```python
from build123d import *

# Parameters (mm, degrees)
SKETCH1_W           = 40
SKETCH1_H           = 40
BOSS_EXTRUDE1_DEPTH = 90
SKETCH2_R           = 18.5
CUT_EXTRUDE1_DEPTH  = 45
SKETCH3_R           = 16.5
CUT_EXTRUDE2_DEPTH  = 41
SKETCH4_W           = 40
SKETCH4_H           = 40
CUT_EXTRUDE3_DEPTH  = 21
SKETCH6_W           = 20
SKETCH6_H           = 15
CUT_EXTRUDE4_DEPTH  = 83.225300243
SKETCH8_W           = 20
SKETCH8_H           = 15
CUT_EXTRUDE5_DEPTH  = 83.225300243
SKETCH16_W          = 40
SKETCH16_H          = 4
BOSS_EXTRUDE3_DEPTH = 8
SKETCH17_W          = 40
SKETCH17_H          = 4
BOSS_EXTRUDE4_DEPTH = 8
SKETCH18_W          = 56
SKETCH18_H          = 4
BOSS_EXTRUDE5_DEPTH = 8
SKETCH19_W          = 56
SKETCH19_H          = 4
BOSS_EXTRUDE6_DEPTH = 8
SKETCH20_R          = 1.5
CUT_EXTRUDE9_DEPTH  = 54.853969213


with BuildPart() as part:
    # Sketch1 → Boss-Extrude1 (new body)
    with BuildSketch(Plane(origin=(0, 0, 0), x_dir=(1, 0, 0), z_dir=(0, 1, 0))):
        Rectangle(SKETCH1_W, SKETCH1_H)
    extrude(amount=BOSS_EXTRUDE1_DEPTH)

    # Sketch2 → Cut-Extrude1 (cut)
    with BuildSketch(Plane(origin=(0, 90, 0), x_dir=(1, 0, 0), z_dir=(0, 1, 0))):
        with Locations(Location((0, 0, 0), (0, 0, 270))):
            Circle(SKETCH2_R)
    extrude(amount=-CUT_EXTRUDE1_DEPTH, mode=Mode.SUBTRACT)

    # Sketch3 → Cut-Extrude2 (cut)
    with BuildSketch(Plane(origin=(0, 45, 0), x_dir=(1, 0, 0), z_dir=(0, 1, 0))):
        with Locations(Location((0, 0, 0), (0, 0, 270))):
            Circle(SKETCH3_R)
    extrude(amount=-CUT_EXTRUDE2_DEPTH, mode=Mode.SUBTRACT)

    # Sketch4 → Cut-Extrude3 (cut)
    with BuildSketch(Plane(origin=(0, 90, 0), x_dir=(1, 0, 0), z_dir=(0, 1, 0))):
        Rectangle(SKETCH4_W, SKETCH4_H)
    extrude(amount=-CUT_EXTRUDE3_DEPTH, mode=Mode.SUBTRACT)

    # Sketch6 → Cut-Extrude4 (cut, through all)
    with BuildSketch(Plane.XY.offset(20)):
        with Locations((0, 15)):
            Rectangle(SKETCH6_W, SKETCH6_H)
    extrude(amount=-CUT_EXTRUDE4_DEPTH, mode=Mode.SUBTRACT)

    # Sketch8 → Cut-Extrude5 (cut, through all)
    with BuildSketch(Plane.ZY.offset(20)):
        with Locations((0, 15)):
            Rectangle(SKETCH8_W, SKETCH8_H)
    extrude(amount=-CUT_EXTRUDE5_DEPTH, mode=Mode.SUBTRACT)

    # Sketch16 → Boss-Extrude3 (add)
    with BuildSketch(Plane.XY.offset(20)):
        with Locations((0, 30.5)):
            Rectangle(SKETCH16_W, SKETCH16_H)
    extrude(amount=BOSS_EXTRUDE3_DEPTH)

    # Sketch17 → Boss-Extrude4 (add)
    with BuildSketch(Plane(origin=(0, 0, -20), x_dir=(-1, 0, 0), z_dir=(0, 0, -1))):
        with Locations((0, 30.5)):
            Rectangle(SKETCH17_W, SKETCH17_H)
    extrude(amount=BOSS_EXTRUDE4_DEPTH)

    # Sketch18 → Boss-Extrude5 (add)
    with BuildSketch(Plane(origin=(20, 0, 0), x_dir=(0, 0, -1), z_dir=(1, 0, 0))):
        with Locations((0, 30.5)):
            Rectangle(SKETCH18_W, SKETCH18_H)
    extrude(amount=BOSS_EXTRUDE5_DEPTH)

    # Sketch19 → Boss-Extrude6 (add)
    with BuildSketch(Plane.ZY.offset(20)):
        with Locations((0, 30.5)):
            Rectangle(SKETCH19_W, SKETCH19_H)
    extrude(amount=BOSS_EXTRUDE6_DEPTH)

    # Sketch20 → Cut-Extrude9 (cut, through all)
    with BuildSketch(Plane(origin=(0, 32.5, 0), x_dir=(1, 0, 0), z_dir=(0, 1, 0))):
        with Locations(Location((-24, 24, 0), (0, 0, 270))):
            Circle(SKETCH20_R)
        with Locations(Location((24, 24, 0), (0, 0, 270))):
            Circle(SKETCH20_R)
        with Locations(Location((24, -24, 0), (0, 0, 270))):
            Circle(SKETCH20_R)
        with Locations(Location((-24, -24, 0), (0, 0, 270))):
            Circle(SKETCH20_R)
    extrude(amount=-CUT_EXTRUDE9_DEPTH, mode=Mode.SUBTRACT)


solid = part.part
```
Input: part model. Units: mm. Frame: model coordinates. A direction names the side the tool comes from. Give positions to 0.01 mm unless a question says otherwise; leave off trailing zeros. Order: outer loops, then holes, each group sorted by start corner. A loop starts at its lowest first (then second) coordinate and runs counter-clockwise, first axis right, second up. Notation, with made-up numbers: M 78.25,74 L 118.25,74 A14 cw 118.25,82 Z; hole C 73,-24 d9. An arc over 180 degrees is marked long. Return JSON: item names as keys, results as strings.
Item 1: Cut plane C-C (y = 30.5). Return loops of the section in (x, z), then the cut area to 3 significant figures.
Solutions:
{"outline": "M -28,-28 L 28,-28 L 28,28 L -28,28 Z; hole C -24,-24 d3; hole C -24,24 d3; hole C 0,0 d33; hole C 24,-24 d3; hole C 24,24 d3", "area": "2,250 mm^2"}
Item 2: Ray query, probe 1 along X at (y, z) = (31.65, -24); probe 2 along Y at (x, z) = (9.5, -18); probe 3 along Z at (x, y) = (0, 27). Return the intervals inside material, ascending.
Solutions:
{"probe 1": "-28 to -25.5, -22.5 to 22.5, 25.5 to 28", "probe 2": "0 to 7.5, 22.5 to 69", "probe 3": "-20 to -16.5, 16.5 to 20"}
Item 3: Cut plane A-A (x = 24). Return loops of the section in (y, z), then the cut area to 3 significant figures.
Solutions:
{"outline": "M 28.5,-28 L 32.5,-28 L 32.5,-25.5 L 28.5,-25.5 Z; M 28.5,-22.5 L 32.5,-22.5 L 32.5,22.5 L 28.5,22.5 Z; M 28.5,25.5 L 32.5,25.5 L 32.5,28 L 28.5,28 Z", "area": "200 mm^2"}
Item 4: Access query for faces 1 (the flat face through (-17, 15, -10)), 2 (the flat face through (-20, 24, 0)), 3 (the flat face through (0, 22.5, -17)), 4 (the flat face through (0, 50, 20)). Directions: +Z, -Z, +X, -X, +Y, -Y. A direction counts if a zero-diameter tool reaches every point of the face in a straight line with its end or side. Return the directions, or none.
Solutions:
{"face 1": "+X, -X", "face 2": "+Z, -Z, -X, -Y", "face 3": "+Z, -Z", "face 4": "+Z, +X, -X, +Y"}
Item 5: Cut plane D-D (y = 17.5). Return loops of the section in (x, z), then the cut area to 3 significant figures.
Solutions:
{"outline": "M -20,-20 L -10,-20 L -10,-13.12 A16.5 cw -13.12,-10 L -20,-10 Z; M -20,10 L -13.12,10 A16.5 cw -10,13.12 L -10,20 L -20,20 Z; M 10,-20 L 20,-20 L 20,-10 L 13.12,-10 A16.5 cw 10,-13.12 Z; M 10,13.12 A16.5 cw 13.12,10 L 20,10 L 20,20 L 10,20 Z", "area": "379 mm^2"}
Item 6: Pull-direction query (Z, two-part tool) for faces 5 (the flat face through (0, 45, -17)), 6 (the flat face through (20, 24, 0)), 7 (the flat face through (0, 24, 20)), 8 (the cylindrical face through (0.725, 29.343, -16.484)); classes: +Z half, -Z half, draft (parallel to the pull), parting line (faces both ways), or undercut.
Solutions:
{"face 5": "undercut", "face 6": "draft", "face 7": "+Z half", "face 8": "undercut"}
Item 7: First-contact query: P1, Ø18, axis at x = 4.5, y = 51, coming from the -Z side; P2, Ø3.5, axis at y = 18.5, z = -18, coming from the -X side; P3, Ø3.5, axis at x = 18, z = 1.5, coming from the +Y side; P4, Ø4, axis at x = -15.5, z = -1.5, coming from the +Y side. Flat tips, straight axial feed; report the tip coordinate or a pass-through.
Solutions:
{"P1": "z = -20", "P2": "x = -20", "P3": "y = 69", "P4": "y = 45"}
Item 8: Cut plane B-B (z = 0). Return loops of the section in (x, y).
Solutions:
{"outline": "M -28,28.5 L -20,28.5 L -20,22.5 L -16.5,22.5 L -16.5,45 L -18.5,45 L -18.5,69 L -20,69 L -20,32.5 L -28,32.5 Z; M -20,0 L 20,0 L 20,7.5 L 16.5,7.5 L 16.5,4 L -16.5,4 L -16.5,7.5 L -20,7.5 Z; M 16.5,22.5 L 20,22.5 L 20,28.5 L 28,28.5 L 28,32.5 L 20,32.5 L 20,69 L 18.5,69 L 18.5,45 L 16.5,45 Z"}
